Can you work these out from the model? Positions are in its coordinate system, mm. A direction names the side the tool comes from. Give positions to 0.01 mm unless a question says otherwise; leave off trailing zeros. Order: outer loops, then holes, each group sorted by start corner. A loop starts at its lowest first (then second) coordinate and runs counter-clockwise, first axis right, second up. Notation, with made-up numbers: M 31,47.25 L 81,47.25 A6 ccw 81,52.25 Z; hole C -11,84 d9. An arc over 180 degrees is marked long. Use one line per item in the form item = value. Start each with the question number.
1. I need wall thicknesses on L1, parallel to X at y = -0.5, z = 2.5; L2, parallel to X at y = 9.5, z = -8; L3, parallel to Y at x = -47.5, z = 31.5. Which ranges of each line are inside material? Lowest first, please.
2. For faces 5 (the face through (0, 11.214, -12)), 6 (the face through (-2.1, 4.65, -17.97)), which set-ups out of +Z, -Z, +X, -X, +Y, -Y let a thin tool reach every point of the face, with its end or its side?
3. Will these pins go through, and if not, where does the flat tip stop? P1, Ø2, axis at x = 15, y = 5, coming from the +Z side; P2, Ø1.5, axis at x = 0, y = 1, coming from the +Z side; P3, Ø15, axis at x = 25.5, z = 23.5, coming from the +Y side.
4. I want a section at A-A, the plane y = 6.75. List the corners of the cut face in (x, z) for me.
5. We'd pull the mould along X, two halves only. Please class faces 1 (the face through (26.32, 2.07, 19.47)), 2 (the face through (-13, -1.486, 7)), 3 (the face through (30.497, 2.066, 13.385)), 4 (the face through (-25.61, 2.07, 18.76)): +X half, -X half, draft (parallel to the pull), parting line (faces both ways), or undercut.
```python
from build123d import *

# Parameters (mm, degrees)
BOSS_EXTRUDE1_DEPTH = 2.54
FILLET4_R           = 2.54
SKETCH2_R           = 3.175
BOSS_EXTRUDE2_DEPTH = 6.35
FILLET5_R           = 1.27
SCALE1_SCALE        = 2


with BuildPart() as part:
    # Sketch1 → Boss-Extrude1 (new body)
    with BuildSketch(Plane(origin=(0, 0, 0), x_dir=(1, 0, 0), z_dir=(0, 1, 0))):
        with BuildLine():
            ThreePointArc((1.796051224, -1.796051224), (2.54, 0), (1.796051224, 1.796051224))
            ThreePointArc((1.796051224, 1.796051224), (0, 2.54), (-1.796051224, 1.796051224))
            ThreePointArc((-1.796051224, 1.796051224), (-2.54, 0), (-1.796051224, -1.796051224))
            Line((-1.796051224, -1.796051224), (0, -3.592102448))
            Line((0, -3.592102448), (1.796051224, -1.796051224))
        make_face()
        with BuildLine():
            Line((28.736819587, -25.144717139), (1.796051224, 1.796051224))
            ThreePointArc((1.796051224, 1.796051224), (2.54, 0), (1.796051224, -1.796051224))
            Line((1.796051224, -1.796051224), (0, -3.592102448))
            Line((0, -3.592102448), (25.144717139, -28.736819587))
            ThreePointArc((25.144717139, -28.736819587), (28.736819587, -28.736819587), (28.736819587, -25.144717139))
        make_face()
        with BuildLine():
            ThreePointArc((-1.796051224, -1.796051224), (-2.54, 0), (-1.796051224, 1.796051224))
            Line((-1.796051224, 1.796051224), (-28.736819587, -25.144717139))
            ThreePointArc((-28.736819587, -25.144717139), (-28.736819587, -28.736819587), (-25.144717139, -28.736819587))
            Line((-25.144717139, -28.736819587), (0, -3.592102448))
            Line((0, -3.592102448), (-1.796051224, -1.796051224))
        make_face()
    extrude(amount=BOSS_EXTRUDE1_DEPTH)

    # Fillet4
    fillet4_edges = [part.edges().sort_by_distance(p)[0] for p in [
        (-28.736819587, 2.54, 28.736819587),
        (-15.266435406, 2.54, 11.674332957),
        (0, 2.54, -2.54),
        (15.266435406, 2.54, 11.674332957),
        (28.736819587, 2.54, 28.736819587),
        (12.572358569, 2.54, 16.164461018),
        (-12.572358569, 2.54, 16.164461018),
    ]]
    fillet(fillet4_edges, radius=FILLET4_R - 0.0001)  # a hair under: the kernel refuses the full size

    # Sketch2 → Boss-Extrude2 (add)
    with BuildSketch(Plane(origin=(0, 0, 0), x_dir=(1, 0, 0), z_dir=(0, 1, 0))):
        with Locations(Location((0, 0, 0), (0, 0, 171.869897646))):
            Circle(SKETCH2_R)
    extrude(amount=BOSS_EXTRUDE2_DEPTH)

    # Fillet5
    fillet5_edges = [part.edges().sort_by_distance(p)[0] for p in [
        (3.143089642, 6.35, 0.449012806),
    ]]
    fillet(fillet5_edges, radius=FILLET5_R)


with BuildPart() as part_1:
    # Scale1: scaled about (-2.1e-08, 1.486347435, 11.976765816)
    add(part.part.scale(SCALE1_SCALE).moved(Location((2.1e-08, -1.486347435, -11.976765816))))


solid = part_1.part
```
Check result:
q1.L1 = -21.52 to -7.43, 7.43 to 21.52
q1.L2 = -4.77 to 4.77
q1.L3 = -1.49 to 2.72
q2.face_5 = +Z, -Z, +X, -X, +Y
q2.face_6 = +Y
q3.P1 = through
q3.P2 = -4.79
q3.P3 = 3.59
q4.outline = C 0,-11.98 d12.7
q5.face_1 = undercut
q5.face_2 = draft
q5.face_3 = +X half
q5.face_4 = undercut
